Autodesk Inventor part; units mm, degrees
ref_plane "YZ Plane" through (0, 0, 0) normal (1, 0, 0) x (0, 1, 0)
ref_plane "XZ Plane" through (0, 0, 0) normal (0, 1, 0) x (-1, 0, 0)
ref_plane "XY Plane" through (0, 0, 0) normal (0, 0, 1) x (1, 0, 0)
sketch "Náčrt1" plane through (0, 0, 0) normal (0, 1, 0) x (-1, 0, 0)
  line L0 (0, 0) -> (50, 0)
  line L1 (50, 0) -> (50, -69)
  line L2 (50, -69) -> (16, -69)
  line L3 (16, -69) -> (16, -81)
  line L4 (16, -81) -> (25.25, -81)
  line L5 (25.25, -81) -> (25.25, -69)
  line L6 (25.25, -81) -> (25.25, -91.25)
  line L7 (25.25, -91.25) -> (25.25, -100)
  line L8 (25.25, -100) -> (0, -100)
  line L9 (0, -100) -> (0, -91.25)
  line L10 (0, -91.25) -> (25.25, -91.25)
  line L11 (0, -91.25) -> (0, -85.25)
  line L12 (0, -85.25) -> (16, -85.25)
  line L13 (16, -85.25) -> (16, -81)
  line L14 (0, -85.25) -> (0, 0)
  line L15 (16, -69) -> (16, -57.25)
  line L16 (16, -57.25) -> (0, -57.25)
  line L17 (48, -25) -> (48, -61.5)
  line L18 (48, -61.5) -> (42.5, -61.5)
  line L19 (42.5, -61.5) -> (42.5, -67)
  line L20 (42.5, -67) -> (16, -67)
  line L21 (0, -25) -> (48, -25)
  dimension "d0" = 50
  dimension "d1" = 69
  dimension "d2" = 12
  dimension "d3" = 10.25
  dimension "d4" = 8.75
  dimension "d5" = 25.25
  dimension "d6" = 16
  dimension "d7" = 6
  dimension "d9" = 2
  dimension "d10" = 7.5
  dimension "d11" = 7.5
  dimension "d12" = 28
  dimension "d13" = 25
  dimension "d18" = 2
extrude "Vysunutí1" add sketch "Náčrt1" along normal blind 3 contours L21 L17 L18 L19 L20 L15 L16 L14
extrude "Vysunutí2" add sketch "Náčrt1" along normal blind 1.888 contours L16 L15 L3 L13 L12 L14
extrude "Vysunutí3" add sketch "Náčrt1" along normal blind 22.5 contours L0 L1 L2 L15 L20 L19 L18 L17 L21 L14
extrude "Vysunutí4" add sketch "Náčrt1" along normal blind 17 contours L5 L4 L3 L2 | L10 L7 L8 L9
extrude "Vysunutí15" add sketch "Náčrt1" along normal blind 5 contours L12 L13 L4 L6 L10 L11
sketch "Náčrt15" plane through (-48, 3, -61.5) normal (1, 0, 0) x (0, 0, -1)
  line L0 (5.5, 0) -> (5.5, 19.5)
  line L1 (0, 0) -> (0, 19.5)
  line L2 (0, 0) -> (5.5, 0)
  line L3 (5.5, 0) -> (5.5, 7.75)
  line L4 (5.5, 0) -> (5.5, 19.5)
  line L5 (5.5, 7.75) -> (0, 13.25)
  line L6 (0, 0) -> (0, 13.25)
  line L7 (0, 19.5) -> (5.5, 19.5)
  line L8 (0, 0) -> (-36.5, 0)
  point P0 (-61.5, -3)
  point P1 (5.5, 7.75)
  point P2 (2.75, 19.5)
  point P3 (2.75, 10.5)
  dimension "d107" = 45
  dimension "d110" = 9
extrude "Vysunutí14" cut sketch "Náčrt15" along normal up to surface (5.5 mm away) contours L2 L1 L5 L0
sketch "Náčrt2" plane through (-50, 0, -69) normal (-1, 0, 0) x (0, 0, 1)
  line L0 (69, 0) -> (69, 22.5)
  line L1 (69, 0) -> (59, 4.5)
  line L2 (0, 0) -> (69, 0)
  line L3 (44, 0) -> (44, 22.5)
  line L4 (44, 3) -> (44, 22.5)
  line L5 (44, 22.5) -> (44, 25)
  line L6 (44, 25) -> (59, 4.5)
  line L7 (0, 22.5) -> (69, 22.5)
  point P0 (45.8293, 22.5)
  dimension "d23" = 25
  dimension "d24" = 4.5
  dimension "d25" = 10
extrude "Vysunutí5" cut sketch "Náčrt2" against normal through all contours L1 L6 L7 L0
extrude "Vysunutí6" add sketch "Náčrt2" against normal up to surface (50 mm away) contours L7 L5 L6
sketch "Náčrt3" plane through (0, 3, -25) normal (0, 0, -1) x (-1, 0, 0)
  line L0 (23, 15.167) -> (38, 15.167)
  line L1 (38, 15.167) -> (38, 0)
  line L2 (38, 0) -> (23, 0)
  line L3 (23, 0) -> (23, 15.167)
  line L4 (0, 15.167) -> (7.5, 15.167)
  line L5 (7.5, 15.167) -> (7.5, 0)
  line L6 (7.5, 0) -> (0, 0)
  line L7 (0, 0) -> (0, 15.167)
  line L8 (50, -3) -> (0, -3)
  dimension "d30" = 15
  dimension "d31" = 7.5
  dimension "d32" = 15.167
  dimension "d33" = 3
  dimension "d34" = 15.5
extrude "Vysunutí7" cut sketch "Náčrt3" against normal blind 9
sketch "Náčrt7" plane through (-48, 3, -61.5) normal (1, 0, 0) x (0, 0, -1)
  line L0 (-51.5, 1.5) -> (-36.5, 22)
  line L1 (-36.5, 15.167) -> (-36.5, 0)
  line L2 (-36.5, 0) -> (-44.5, 0)
  line L3 (-36.5, 0) -> (-45.5, 0)
  line L4 (-44.5, 0) -> (-44.5, 6.833)
  line L5 (-44.5, 6.833) -> (-36.5, 17.7664)
  line L6 (-36.5, 17.7664) -> (-36.5, 0)
  point P0 (-61.5, -3)
  point P1 (-38.3293, 19.5)
  point P2 (-44.5, 0)
  point P3 (-36.5, 2)
  point P4 (-36.5, 2)
  dimension "d45" = 8
  dimension "d46" = 2.5
extrude "Vysunutí9" cut sketch "Náčrt7" along normal through all
sketch "Náčrt11" plane through (-48, 22.5, -25) normal (0, 0, -1) x (-1, 0, 0)
  line L0 (2, -18) -> (2, 2.5)
  line L1 (2, 2.5) -> (0, 2.5)
  line L2 (0, 2.5) -> (0, 1.5)
  line L3 (0, 1.5) -> (2, 1.5)
  point P0 (-48, -22.5)
  point P1 (0, 0)
  point P2 (-2, 0)
  dimension "d69" = 1
extrude "Vysunutí13" add sketch "Náčrt11" along normal blind 1
sketch "Náčrt12" plane through (0, 22.5, 0) normal (0, 1, 0) x (1, 0, 0)
  line L0 (-16, 69) -> (-50, 69)
  line L1 (-50, 69) -> (-50, 23.1707)
  point P0 (0, 0)
  point P1 (-46.25, 65.25)
  point P2 (-50, 25)
  dimension "d75" = 3.75
  dimension "d76" = 3.75
hole "Díra1" at (-46.25, 22.5, -65.25) direction (0, -1, 0) diameter 3 depth 6
sketch "Náčrt13" plane through (0, 17, 0) normal (0, 1, 0) x (1, 0, 0)
  line L0 (-16, 81) -> (-25.25, 81)
  line L1 (-25.25, 81) -> (-25.25, 69)
  point P0 (0, 0)
  point P1 (-20.625, 75)
  dimension "d84" = 6
  dimension "d85" = 4.625
hole "Díra2" at (-20.625, 17, -75) direction (0, -1, 0) diameter 3 depth 6
sketch "Náčrt14" plane through (0, 17, 0) normal (0, 1, 0) x (1, 0, 0)
  line L0 (-25.25, 100) -> (-25.25, 91.25)
  line L1 (0, 100) -> (-25.25, 100)
  point P0 (0, 0)
  point P1 (-20.125, 95.5)
  dimension "d93" = 5.125
  dimension "d101" = 4.5
hole "Díra3" at (-20.125, 17, -95.5) direction (0, -1, 0) diameter 3 depth 6
fillet "Zaoblení1" radius 3 2 edges at (-16, 2.444, -57.25) (-16, 3.444, -85.25)
fillet "Zaoblení2" radius 1 2 edges at (-42.5, 19.375, -61.5) (-50, 11.25, -69)
fillet "Zaoblení3" radius 5 1 edges at (-25.25, 8.5, -100)
mirror "Zrcadlit1" about plane through (0, 0, -25) normal (1, 0, 0)
sketch "Náčrt16" plane through (0, 1.888, 0) normal (0, 1, 0) x (1, 0, 0)
  line L0 (-9.4, 73.625) -> (-13.4, 73.625)
  line L1 (-13.4, 73.625) -> (-13.4, 78.375)
  line L2 (-13.4, 78.375) -> (-9.4, 78.375)
  line L3 (-9.4, 78.375) -> (-9.4, 73.625)
  line L4 (-16, 69) -> (-16, 81)
  line L5 (-13, 85.25) -> (13, 85.25)
  line L6 (13.75, 73.625) -> (9.75, 73.625)
  line L7 (9.75, 73.625) -> (9.75, 78.375)
  line L8 (9.75, 78.375) -> (13.75, 78.375)
  line L9 (13.75, 78.375) -> (13.75, 73.625)
  line L10 (16, 69) -> (16, 81)
  point P0 (0, 0)
  dimension "d128" = 4
  dimension "d129" = 4.75
  dimension "d130" = 2.6
  dimension "d131" = 6.875
  dimension "d134" = 2.25
extrude "Vysunutí16" cut sketch "Náčrt16" against normal through all
sketch "Náčrt17" plane through (0, 3, 0) normal (0, 1, 0) x (1, 0, 0)
  line L0 (-48, 17) -> (-38, 17)
  line L1 (-48, 17) -> (-48, 67)
  line L2 (48, 17) -> (38, 17)
  line L3 (48, 17) -> (48, 67)
  line L4 (-39.4, 19.625) -> (-43.4, 19.625)
  line L5 (-43.4, 19.625) -> (-43.4, 24.375)
  line L6 (-43.4, 24.375) -> (-39.4, 24.375)
  line L7 (-39.4, 24.375) -> (-39.4, 19.625)
  line L8 (42.75, 19.625) -> (38.75, 19.625)
  line L9 (38.75, 19.625) -> (38.75, 24.375)
  line L10 (38.75, 24.375) -> (42.75, 24.375)
  line L11 (42.75, 24.375) -> (42.75, 19.625)
  point P0 (0, 0)
  point P1 (-41.4, 19.625)
  point P2 (40.75, 19.625)
  dimension "d137" = 4
  dimension "d138" = 4.75
  dimension "d139" = 4.6
  dimension "d143" = 2.625
  dimension "d144" = 5.25
  dimension "d146" = 2.625
extrude "Vysunutí17" cut sketch "Náčrt17" against normal through all
sketch "Náčrt18" plane through (0, 3, 0) normal (0, 1, 0) x (1, 0, 0)
  circle A0 centre (39.25, 59) radius 3.75
  circle A1 centre (-40.5, 29) radius 3.75
  line L0 (42.5, 67) -> (16, 67)
  line L1 (48, 25) -> (48, 61.5)
  line L2 (-48, 17) -> (-38, 17)
  line L3 (-48, 17) -> (-48, 67)
  point P0 (0, 0)
  dimension "d149" = 7.5
  dimension "d150" = 8
  dimension "d151" = 8.75
  dimension "d152" = 12
  dimension "d153" = 7.5
extrude "Vysunutí18" add sketch "Náčrt18" along normal blind 5
sketch "Náčrt19" plane through (39.25, 8, -59) normal (0, 1, 0) x (1, 0, 0)
  circle A0 centre (0, 0) radius 3.75
  point P0 (-39.25, -59)
hole "Díra4" at (39.25, 8, -59) direction (0, -1, 0) diameter 3 depth 6
sketch "Náčrt20" plane through (-40.5, 8, -29) normal (0, 1, 0) x (1, 0, 0)
  circle A0 centre (0, 0) radius 3.75
  point P0 (40.5, -29)
hole "Díra5" at (-40.5, 8, -29) direction (0, -1, 0) diameter 3 depth 6
properties part number "Sumec_telo_V4.1"
Input: part model. Units: mm. Frame: model coordinates. A direction names the side the tool comes from. Coordinates: 2 decimals unless noted, no trailing zeros. Loops run counter-clockwise (first coordinate to the right, second up) from the corner with the lowest first, then second, coordinate; pieces in that order, holes last. Notation, with made-up numbers: M 15,32 L 22,32 A21 ccw 22,57 Z; hole C -17,75 d7. An arc over 180 degrees is marked long. Answer in a Markdown table with one row per item.
1. Draft query along X for faces 1 (the flat face through (-23, 12.2, -18.5)), 2 (the flat face through (0, 5, -87)), 3 (the flat face through (-50, 10, -41)). Return one class per face: pulls with the +X half, pulls with the -X half, needs draft (parallel to the pull), parting line crosses it, or undercut.
Response:
| item | result |
|---|---|
| face 1 | undercut |
| face 2 | needs draft |
| face 3 | pulls with the -X half |
2. Reachability of faces 4 (the flat face through (-38, 12.3, -18.5)), 5 (the flat face through (0, 3, -85.25)), 6 (the flat face through (31, 18.167, -22)) from +Z, -Z, +X, -X, +Y, -Y: full face, straight path, thin tool, end or side. Return the list, or none.
Response:
| item | result |
|---|---|
| face 4 | none |
| face 5 | +Y |
| face 6 | +Z |
3. Section A-A, the plane x = 6. Output: boundary loops of the cut face in (y, z).
Response:
| item | result |
|---|---|
| outline | M 0,-100 L 17,-100 L 17,-91.25 L 5,-91.25 L 5,-85.25 L 1.89,-85.25 L 1.89,-57.25 L 3,-57.25 L 3,-16 L 12.7,-16 L 4.5,-10 L 0,0 Z; M 18.17,-23.1 L 20.77,-25 L 25,-25 L 18.17,-20 Z |
4. Section C-C, the plane z = -43. Output: boundary loops of the cut face in (x, y), then the cut area to 3 significant figures.
Response:
| item | result |
|---|---|
| outline | M -50,0 L 50,0 L 50,22.5 L 48,22.5 L 48,3 L -48,3 L -48,22.5 L -50,22.5 Z |
| area | 378 mm2 |
5. Section D-D, the plane x = -46.25. Output: boundary loops of the cut face in (y, z), then the cut area to 3 significant figures.
Response:
| item | result |
|---|---|
| outline | M 0,-69 L 22.5,-69 L 22.5,-66.75 L 16.5,-66.75 L 16.5,-63.75 L 22.5,-63.75 L 22.5,-61.5 L 16.25,-61.5 L 10.75,-67 L 3,-67 L 3,-17 L 9.83,-17 L 20.77,-25 L 25,-25 L 4.5,-10 L 0,0 Z |
| area | 348 mm2 |
6. First-contact query: pin 1 (2.5 mm diameter, centred on x = 20.625, z = -75, fed in from -Y); pin 2 (5 mm diameter, centred on x = 34, y = 9.5, fed in from -Z); pin 3 (11 mm diameter, centred on x = 26, y = 16, fed in from -Z); pin 4 (10 mm diameter, centred on x = -5, z = -34.5, fed in from +Y). Flat tips, straight axial feed; report the tip coordinate or a pass-through.
Response:
| item | result |
|---|---|
| pin 1 | stops at y = 0 |
| pin 2 | stops at z = -69 |
| pin 3 | stops at z = -99.99 |
| pin 4 | stops at y = 3 |
7. Section B-B, the plane z = -75. Output: boundary loops of the cut face in (x, y) (3 decimals).
Response:
| item | result |
|---|---|
| outline | M -25.25,0 L -13.4,0 L -13.4,1.888 L -16,1.888 L -16,17 L -19.125,17 L -19.125,11 L -22.125,11 L -22.125,17 L -25.25,17 Z; M -9.4,0 L 9.75,0 L 9.75,1.888 L -9.4,1.888 Z; M 13.75,0 L 25.25,0 L 25.25,17 L 22.125,17 L 22.125,11 L 19.125,11 L 19.125,17 L 16,17 L 16,1.888 L 13.75,1.888 Z |
8. Material intervals for line 1 (X direction, y = 13.2, z = -75) (3 decimals); line 2 (X direction, y = 14.75, z = -95.5) (3 decimals); line 3 (X direction, y = 4.75, z = -29), sorted ascending.
Response:
| item | result |
|---|---|
| line 1 | x = -25.25 to -22.125, -19.125 to -16, 16 to 19.125, 22.125 to 25.25 |
| line 2 | x = -25.225 to -21.625, -18.625 to 18.625, 21.625 to 25.225 |
| line 3 | x = -50 to -48, -44.25 to -42, -39 to -36.75, 48 to 50 |
